Design review of the part built by this model. Coordinates are the model's own, in mm. Coordinates: 2 decimals unless noted, no trailing zeros. Write each loop counter-clockwise with the first axis right and the second up, starting at its lowest first coordinate (ties: lowest second). Pieces come first, ordered by that corner, then holes. Notation, with made-up numbers: (81, 27) - (111, 27) arc R11 cw to (111, 43) - close; hole circle Ø9 at (7, 38.25). An arc over 180 degrees is marked (long way). One line per item, written item: value.
from build123d import *

# Parameters (mm, degrees)
EXTRUDE1_DEPTH  = 100
SKETCH2_R       = 3
EXTRUDE2_DEPTH  = 3.5
SKETCH_R        = 1.75
EXTRUDE3_DEPTH  = 7
LPATTERN1_COUNT = 30
LPATTERN1_PITCH = 20


with BuildPart() as part:
    # Sketch1 → Extrude1 (new body)
    with BuildSketch(Plane.XY):
        with BuildLine():
            Line((-4.5, -3), (4.5, -3))
            Line((4.5, -3), (4.5, 0))
            ThreePointArc((4.5, 0), (3.93077967, 0.177814974), (3.563991137, 0.648023568))
            Line((3.563991137, 0.648023568), (3.235073025, 0.648023568))
            Line((3.235073025, 0.648023568), (3.235073025, 1.351976432))
            Line((3.235073025, 1.351976432), (3.563991137, 1.351976432))
            ThreePointArc((3.563991137, 1.351976432), (3.93077967, 1.822185026), (4.5, 2))
            Line((4.5, 2), (4.5, 3))
            Line((4.5, 3), (-4.5, 3))
            Line((-4.5, 3), (-4.5, 2))
            ThreePointArc((-4.5, 2), (-3.93077967, 1.822185026), (-3.563991137, 1.351976432))
            Line((-3.563991137, 1.351976432), (-3.235073025, 1.351976432))
            Line((-3.235073025, 1.351976432), (-3.235073025, 0.648023568))
            Line((-3.235073025, 0.648023568), (-3.563991137, 0.648023568))
            ThreePointArc((-3.563991137, 0.648023568), (-3.93077967, 0.177814974), (-4.5, 0))
            Line((-4.5, 0), (-4.5, -3))
        make_face()
    extrude(amount=EXTRUDE1_DEPTH)

    # Sketch2 → Extrude2 (cut)
    with BuildSketch(Plane(origin=(0, 3, 0), x_dir=(1, 0, 0), z_dir=(0, 1, 0))):
        with Locations((0, -5)):
            Circle(SKETCH2_R)
    extrude2 = extrude(amount=-EXTRUDE2_DEPTH, mode=Mode.SUBTRACT)

    # Sketch → Extrude3 (cut, through all)
    with BuildSketch(Plane(origin=(0, 3, 0), x_dir=(1, 0, 0), z_dir=(0, 1, 0))):
        with Locations((0, -5)):
            Circle(SKETCH_R)
    extrude3 = extrude(amount=-EXTRUDE3_DEPTH, mode=Mode.SUBTRACT)

    # LPattern1: Extrude2, Extrude3 ×30
    with Locations(*[(0, 0, i * LPATTERN1_PITCH) for i in range(1, LPATTERN1_COUNT)]):
        add(extrude2, mode=Mode.SUBTRACT)
        add(extrude3, mode=Mode.SUBTRACT)


solid = part.part
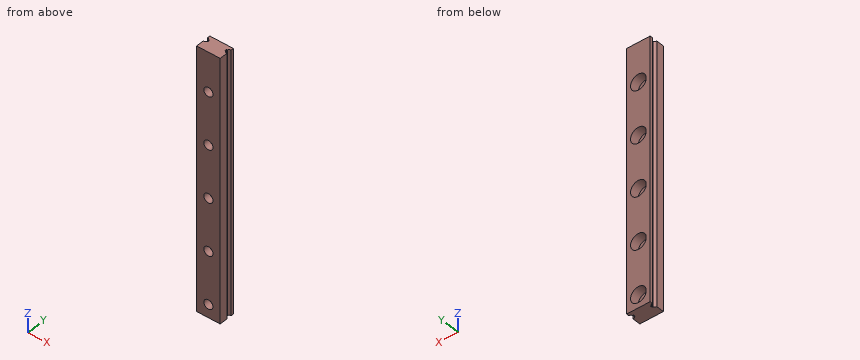
1. Wall thickness on line 1 along Z through (x, y) = (0, -1.4); line 2 along Z through (x, y) = (0, 0.9); line 3 along X through (y, z) = (2.15, 25): over which ranges is each line inside the solid? List them lowest first.
Answer block:
line 1: z = 0 to 3.25, 6.75 to 23.25, 26.75 to 43.25, 46.75 to 63.25, 66.75 to 83.25, 86.75 to 100
line 2: z = 0 to 2, 8 to 22, 28 to 42, 48 to 62, 68 to 82, 88 to 100
line 3: x = -4.5 to -3, 3 to 4.5
2. Consider section B-B, the plane z = 45. Write out the cut boundary in (x, y), then the cut area to 3 significant figures.
Answer block:
outline: (-4.5, -3) - (-1.75, -3) - (-1.75, -0.5) - (-3, -0.5) - (-3, 3) - (-4.5, 3) - (-4.5, 2) arc R1 cw to (-3.56, 1.35) - (-3.24, 1.35) - (-3.24, 0.65) - (-3.56, 0.65) arc R1 cw to (-4.5, 0) - close; (1.75, -3) - (4.5, -3) - (4.5, 0) arc R1 cw to (3.56, 0.65) - (3.24, 0.65) - (3.24, 1.35) - (3.56, 1.35) arc R1 cw to (4.5, 2) - (4.5, 3) - (3, 3) - (3, -0.5) - (1.75, -0.5) - close
area: 20.7 mm^2
3. Insertion check: pin 1 Ø0.8 at (y, z) = (1, 32.5) entering from +X; pin 2 Ø2 at (x, z) = (0, 85) entering from +Y; pin 3 Ø3 at (x, z) = (1, 5.5) entering from +Y. Each pin has a flat end and moves straight along its axis. Give the tip position at first contact, or say it passes through.
Answer block:
pin 1: stops at x = 3.58
pin 2: passes through
pin 3: stops at y = -0.5
4. Consider section D-D, the plane x = 0. Give the number of separate pieces and of enclosed holes in the cut face, then the cut area to 3 significant figures.
Answer block:
separate pieces: 6
enclosed holes: 0
area: 451 mm^2
5. Consider section A-A, the plane y = -1.65. Write out the cut boundary in (x, z).
Answer block:
outline: (-4.5, 0) - (4.5, 0) - (4.5, 100) - (-4.5, 100) - close; hole circle Ø3.5 at (0, 5); hole circle Ø3.5 at (0, 25); hole circle Ø3.5 at (0, 45); hole circle Ø3.5 at (0, 65); hole circle Ø3.5 at (0, 85)
6. Consider section C-C, the plane z = 20.5. Write out the cut boundary in (x, y), then the cut area to 3 significant figures.
Answer block:
outline: (-4.5, -3) - (4.5, -3) - (4.5, 0) arc R1 cw to (3.56, 0.65) - (3.24, 0.65) - (3.24, 1.35) - (3.56, 1.35) arc R1 cw to (4.5, 2) - (4.5, 3) - (-4.5, 3) - (-4.5, 2) arc R1 cw to (-3.56, 1.35) - (-3.24, 1.35) - (-3.24, 0.65) - (-3.56, 0.65) arc R1 cw to (-4.5, 0) - close
area: 50.5 mm^2
